```python
from build123d import *

# Parameters (mm, degrees)
F0_W      = 260
F0_H      = 210
F0_W_2    = 40
F0_H_2    = 40
F1_DEPTH  = 20
F1_FACE_W = 260
F1_FACE_H = 20
F2_DEPTH  = 33
F3_W      = 260
F3_H      = 10
F4_DEPTH  = 25
F5_R      = 4.95
F6_DEPTH  = 25
F7_W      = 243
F7_H      = 10
F8_DEPTH  = 25
F9_R      = 4.95
F10_DEPTH = 25
F11_W     = 243
F11_H     = 20
F12_DEPTH = 30
F14_DEPTH = 25
F15_R     = 7.05
F16_DEPTH = 3


with BuildPart() as f1:
    # F0 (on Top) → F1 (new body)
    with BuildSketch(Plane.XY):
        Rectangle(F0_W, F0_H)
        with Locations((-100, -75)):
            Rectangle(F0_W_2, F0_H_2, mode=Mode.SUBTRACT)
        with Locations((-50, -75)):
            Rectangle(F0_W_2, F0_H_2, mode=Mode.SUBTRACT)
        with Locations((-100, -25)):
            Rectangle(F0_W_2, F0_H_2, mode=Mode.SUBTRACT)
        with Locations((-50, -25)):
            Rectangle(F0_W_2, F0_H_2, mode=Mode.SUBTRACT)
        with Locations((0, -75)):
            Rectangle(F0_W_2, F0_H_2, mode=Mode.SUBTRACT)
        with Locations((50, -75)):
            Rectangle(F0_W_2, F0_H_2, mode=Mode.SUBTRACT)
        with Locations((100, -75)):
            Rectangle(F0_W_2, F0_H_2, mode=Mode.SUBTRACT)
        with Locations((0, -25)):
            Rectangle(F0_W_2, F0_H_2, mode=Mode.SUBTRACT)
        with Locations((50, -25)):
            Rectangle(F0_W_2, F0_H_2, mode=Mode.SUBTRACT)
        with Locations((100, -25)):
            Rectangle(F0_W_2, F0_H_2, mode=Mode.SUBTRACT)
        with Locations((-100, 25)):
            Rectangle(F0_W_2, F0_H_2, mode=Mode.SUBTRACT)
        with Locations((-50, 25)):
            Rectangle(F0_W_2, F0_H_2, mode=Mode.SUBTRACT)
        with Locations((-100, 75)):
            Rectangle(F0_W_2, F0_H_2, mode=Mode.SUBTRACT)
        with Locations((-50, 75)):
            Rectangle(F0_W_2, F0_H_2, mode=Mode.SUBTRACT)
        with Locations((0, 25)):
            Rectangle(F0_W_2, F0_H_2, mode=Mode.SUBTRACT)
        with Locations((50, 25)):
            Rectangle(F0_W_2, F0_H_2, mode=Mode.SUBTRACT)
        with Locations((100, 25)):
            Rectangle(F0_W_2, F0_H_2, mode=Mode.SUBTRACT)
        with Locations((0, 75)):
            Rectangle(F0_W_2, F0_H_2, mode=Mode.SUBTRACT)
        with Locations((50, 75)):
            Rectangle(F0_W_2, F0_H_2, mode=Mode.SUBTRACT)
        with Locations((100, 75)):
            Rectangle(F0_W_2, F0_H_2, mode=Mode.SUBTRACT)
    extrude(amount=F1_DEPTH)

    # F1_face (on face) → F2 (join)
    with BuildSketch(Plane(origin=(0, -105, 10), x_dir=(1, 0, 0), z_dir=(0, -1, 0))):
        Rectangle(F1_FACE_W, F1_FACE_H)
    extrude(amount=F2_DEPTH)

    # F3 (on face) → F4 (join)
    with BuildSketch(Plane.XZ.offset(138)):
        with Locations((0, 15)):
            Rectangle(F3_W, F3_H)
    extrude(amount=F4_DEPTH)

    # F5 (on face) → F6 (cut)
    with BuildSketch(Plane.XY.offset(20)):
        with Locations((110, -145.5)):
            Circle(F5_R)
        with Locations((70, -145.5)):
            Circle(F5_R)
        with Locations((30, -145.5)):
            Circle(F5_R)
        with Locations((-10, -145.5)):
            Circle(F5_R)
        with Locations((-50, -145.5)):
            Circle(F5_R)
        with Locations((-90, -145.5)):
            Circle(F5_R)
    extrude(amount=-F6_DEPTH, mode=Mode.SUBTRACT)

    # F7 (on face) → F8 (join)
    with BuildSketch(Plane.YZ.offset(130)):
        with Locations((-16.5, 15)):
            Rectangle(F7_W, F7_H)
    extrude(amount=F8_DEPTH)

    # F9 (on face) → F10 (cut)
    with BuildSketch(Plane.XY.offset(20)):
        with Locations((137.5, -118)):
            Circle(F9_R)
        with Locations((137.5, -78)):
            Circle(F9_R)
        with Locations((137.5, -38)):
            Circle(F9_R)
        with Locations((137.5, 2)):
            Circle(F9_R)
        with Locations((137.5, 42)):
            Circle(F9_R)
        with Locations((137.5, 82)):
            Circle(F9_R)
    extrude(amount=-F10_DEPTH, mode=Mode.SUBTRACT)

    # F11 (on face) → F12 (join)
    with BuildSketch(Plane(origin=(-130, 0, 0), x_dir=(0, -1, 0), z_dir=(-1, 0, 0))):
        with Locations((16.5, 10)):
            Rectangle(F11_W, F11_H)
    extrude(amount=F12_DEPTH)

    # F13 (on face) → F14 (cut)
    with BuildSketch(Plane.XY.offset(20)):
        Polygon((-160, -128), (-160, -138), (-140, -138), (-140, -118), (-150, -118), (-150, -128), align=None)
        Polygon((-140, -58), (-140, -38), (-150, -38), (-150, -48), (-160, -48), (-160, -58), align=None)
        Polygon((-140, 22), (-140, 42), (-150, 42), (-150, 32), (-160, 32), (-160, 22), align=None)
    extrude(amount=-F14_DEPTH, mode=Mode.SUBTRACT)

    # F15 (on face) → F16 (join)
    with BuildSketch(Plane.XY.offset(20)):
        with Locations((100, -116.5)):
            Circle(F15_R)
        with Locations((50, -116.5)):
            Circle(F15_R)
        with Locations((0, -116.5)):
            Circle(F15_R)
        with Locations((-50, -116.5)):
            Circle(F15_R)
        with Locations((-100, -116.5)):
            Circle(F15_R)
    extrude(amount=F16_DEPTH)


solid = f1.part
```
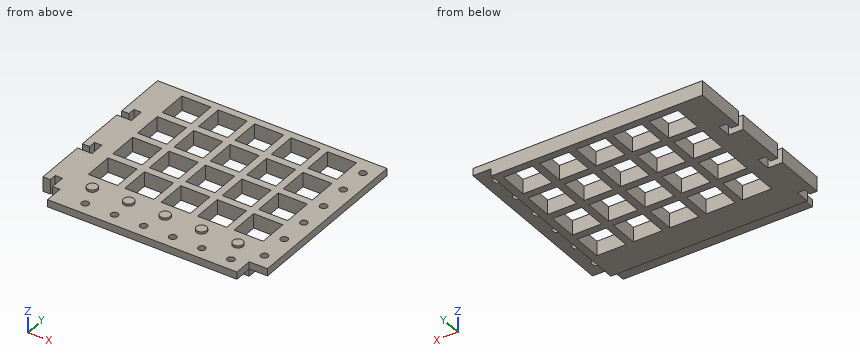
CAD build for the part. Positions are in the model's coordinates, mm. Round coordinates to 2 decimals unless told otherwise and drop trailing zeros. Order: outer loops, then holes, each group sorted by start corner. A loop starts at its lowest first (then second) coordinate and runs counter-clockwise, first axis right, second up.
Q1. Wall check: L1, parallel to Y at x = -102.5, z = 8.5; L2, parallel to X at y = -22, z = 17.25; L3, parallel to Y at x = -50, z = 15. Give the ranges that are in metal, low to high.
Q2. Slice it at D-D (x = 137.5). Write the cut outline in (y, z).
Q3. Slice it at C-C (x = 50). Write the cut outline in (y, z).
Q4. Drop flat-ended pins along their axis: pin 1 (1.5 mm diameter, centred on x = 29.5, y = -14, fed in from -Z); pin 2 (12.5 mm diameter, centred on x = -31.5, y = -154.5, fed in from -Z); pin 3 (13 mm diameter, centred on x = 70, y = -145.5, fed in from +Z); pin 4 (2 mm diameter, centred on x = 57, z = 7, fed in from -Y). Give the stop position or say it passes through.
Q5. Slice it at B-B (y = -145.5). Write the cut outline in (x, z).
Q6. Slice it at A-A (x = -50). State how many separate pieces and enclosed holes the cut face has, and give its area (3 significant figures).
Results below:
1. L1: y = -138 to -95, -55 to -45, -5 to 5, 45 to 55, 95 to 105
1. L2: x = -160 to -120, -80 to -70, -30 to -20, 20 to 30, 70 to 80, 120 to 155
1. L3: y = -163 to -150.45, -140.55 to -95, -55 to -45, -5 to 5, 45 to 55, 95 to 105
2. outline: (-138, 10) - (-122.95, 10) - (-122.95, 20) - (-138, 20) - close; (-113.05, 10) - (-82.95, 10) - (-82.95, 20) - (-113.05, 20) - close; (-73.05, 10) - (-42.95, 10) - (-42.95, 20) - (-73.05, 20) - close; (-33.05, 10) - (-2.95, 10) - (-2.95, 20) - (-33.05, 20) - close; (6.95, 10) - (37.05, 10) - (37.05, 20) - (6.95, 20) - close; (46.95, 10) - (77.05, 10) - (77.05, 20) - (46.95, 20) - close; (86.95, 10) - (105, 10) - (105, 20) - (86.95, 20) - close
3. outline: (-163, 10) - (-138, 10) - (-138, 0) - (-95, 0) - (-95, 20) - (-109.45, 20) - (-109.45, 23) - (-123.55, 23) - (-123.55, 20) - (-163, 20) - close; (-55, 0) - (-45, 0) - (-45, 20) - (-55, 20) - close; (-5, 0) - (5, 0) - (5, 20) - (-5, 20) - close; (45, 0) - (55, 0) - (55, 20) - (45, 20) - close; (95, 0) - (105, 0) - (105, 20) - (95, 20) - close
4. pin 1: stops at z = 0
4. pin 2: stops at z = 10
4. pin 3: stops at z = 20
4. pin 4: stops at y = -138
5. outline: (-130, 10) - (-94.95, 10) - (-94.95, 20) - (-130, 20) - close; (-85.05, 10) - (-54.95, 10) - (-54.95, 20) - (-85.05, 20) - close; (-45.05, 10) - (-14.95, 10) - (-14.95, 20) - (-45.05, 20) - close; (-5.05, 10) - (25.05, 10) - (25.05, 20) - (-5.05, 20) - close; (34.95, 10) - (65.05, 10) - (65.05, 20) - (34.95, 20) - close; (74.95, 10) - (105.05, 10) - (105.05, 20) - (74.95, 20) - close; (114.95, 10) - (130, 10) - (130, 20) - (114.95, 20) - close
6. separate pieces: 6
6. enclosed holes: 0
6. area: 1,850 mm2
